```python
from build123d import *

# Parameters (mm, degrees)
F1_DEPTH = 12.5
F2_R     = 2.05
F3_DEPTH = 25
F4_R     = 1


with BuildPart() as f1:
    # F0 (on Right) → F1 (new body)
    with BuildSketch(Plane.YZ):
        Polygon((-45, 0), (0, 0), (0.431175, -0.097732), (13.965198, -6.56536), (15.689899, -2.956287), (1.133319, 4), (-45, 4), align=None)
    extrude(amount=F1_DEPTH)

    # F2 (on face) → F3 (cut)
    with BuildSketch(Plane(origin=(0, 1.76684, 3.697253), x_dir=(1, 0, 0), z_dir=(0, 0.431175, 0.902268))):
        with Locations((6.25, 7.715588)):
            Circle(F2_R)
    extrude(amount=-F3_DEPTH, mode=Mode.SUBTRACT)

    # F4
    f4_edges = [f1.edges().sort_by_distance(p)[0] for p in [
        (6.25, 1.133319, 4),
        (6.25, -45, 4),
        (0, -21.933341, 4),
        (12.5, -21.933341, 4),
        (12.5, 8.411609, 0.521856),
        (6.25, 15.689899, -2.956287),
        (0, 8.411609, 0.521856),
        (12.5, -22.5, 0),
        (0, -22.5, 0),
        (6.25, -45, 0),
        (12.5, 7.198187, -3.331546),
        (0, 7.198187, -3.331546),
        (6.25, 13.965198, -6.56536),
        (12.5, 0.215588, -0.048866),
        (0, 0.215588, -0.048866),
    ]]
    fillet(f4_edges, radius=F4_R)


solid = f1.part
```
Work out the finished part from the listing and answer in its coordinate system (mm). A direction names the side the tool comes from. Give positions to 0.01 mm unless a question says otherwise; leave off trailing zeros. Loops run counter-clockwise (first coordinate to the right, second up) from the corner with the lowest first, then second, coordinate; pieces in that order, holes last. Notation, with made-up numbers: M 29.5,10.5 L 36.5,10.5 A19 ccw 36.5,40.5 Z; hole C -20,14 d9. An arc over 180 degrees is marked long. One line per item, written item: value. Start each with the question number.
1. Find section B-B (y = -23). Give the vertices of the cut face in (x, z), and give its area (3 significant figures).
2. Find the intervals of material crossed by probe 1 along Z at (x, y) = (4, -5.5); probe 2 along Y at (x, z) = (5.25, -2.25); probe 3 along Y at (x, z) = (3.25, 1.25), in increasing order.
3. Find section C-C (x = 5.5). Give the vertices of the cut face in (y, z), and give its area (3 significant figures).
4. Each of these flat-tipped pins is pushed along its axis until it touches: P1, Ø4, axis at y = -10, z = -1.5, coming from the -X side; P2, Ø1, axis at x = 6.5, y = -32, coming from the -Z side; P3, Ø1, axis at x = 8, z = -2, coming from the -Y side. Where does it stop, or does it pass through?
5. Find section A-A (x = 10.75). Give the vertices of the cut face in (y, z), and give its area (3 significant figures).
6. Which of the six approach directions +Z, -Z, +X, -X, +Y, -Y give full straight-line access (tool end or side, diameter ignored) to faces 1 (the face through (12.199, -22.128, 0.285)), 2 (the face through (6, -22, 0)), 3 (the face through (0.301, -22.128, 0.285))?
Reported:
1. outline: M 0,1 A1 ccw 1,0 L 11.5,0 A1 ccw 12.5,1 L 12.5,3 A1 ccw 11.5,4 L 1,4 A1 ccw 0,3 Z
1. area: 49.1 mm²
2. probe 1: z = 0 to 4
2. probe 2: y = 4.93 to 5.49, 9.46 to 14.21
2. probe 3: y = -45 to 6.89
3. outline: M -45,1 A1 ccw -44,0 L 0,0 L 0.43,-0.1 L 5.28,-2.42 L 7.01,1.19 L 1.34,3.9 A1 ccw 0.91,4 L -44,4 A1 ccw -45,3 Z; M 8.73,-4.06 L 13.06,-6.13 A1 ccw 14.4,-5.66 L 15.26,-3.86 A1 ccw 14.79,-2.53 L 10.45,-0.45 Z
3. area: 229 mm²
4. P1: stops at x = 0.13
4. P2: stops at z = 0
4. P3: stops at y = 3.37
5. outline: M -45,1 A1 ccw -44,0 L 0,0 L 0.43,-0.1 L 13.06,-6.13 A1 ccw 14.4,-5.66 L 15.26,-3.86 A1 ccw 14.79,-2.53 L 1.34,3.9 A1 ccw 0.91,4 L -44,4 A1 ccw -45,3 Z
5. area: 245 mm²
6. face 1: -Z, +X, -Y
6. face 2: -Z, +X, -X, -Y
6. face 3: -Z, -X, -Y
